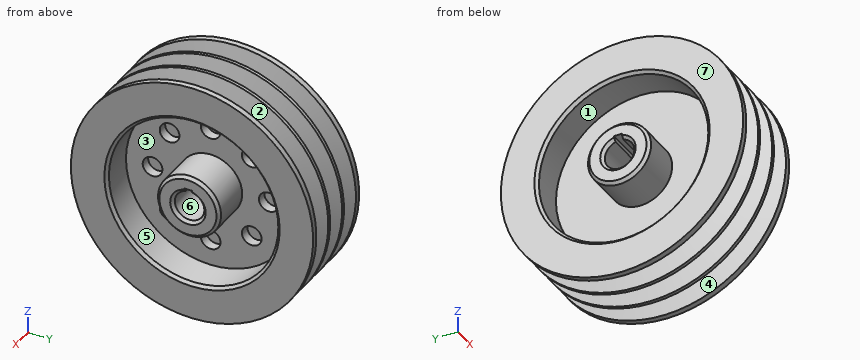
```python
from build123d import *

# Parameters (mm, degrees)
OTHER_START              = -2
OTHER_1_OUTLINE_R        = 10
OTHER_1_DEPTH            = 10
CUT_EXTRUDE_1_DEPTH      = 181.991712517
CUT_EXTRUDE_1_DEPTH_BACK = 181.991712517
SKETCH_4_W               = 24.82633163
SKETCH_4_H               = 8


# Read off the part's stored shape, not the designer's step: 孔1
with BuildPart() as part:
    # 草图1 → 旋转9 (revolve)
    with BuildSketch(Plane.XY, mode=Mode.PRIVATE) as revolve_9_sk:
        Polygon((-47, 15), (47, 15), (50, 18), (50, 29), (47, 32), (8, 32), (8, 86), (39.5, 86), (42.5, 89), (42.5, 123), (36.528653407, 123), (31.178366482, 105.5), (19.821633518, 105.5), (14.471346593, 123), (11.028653407, 123), (5.678366482, 105.5), (-5.678366482, 105.5), (-11.028653407, 123), (-14.471346593, 123), (-19.821633518, 105.5), (-31.178366482, 105.5), (-36.528653407, 123), (-42.5, 123), (-42.5, 89), (-39.5, 86), (-8, 86), (-8, 32), (-47, 32), (-50, 29), (-50, 18), align=None)
    revolve(revolve_9_sk.sketch.rotate(Axis((-111.724769182, 0, 0), (1, 0, 0)), 90), axis=Axis((-111.724769182, 0, 0), (1, 0, 0)))

    # 孔1 outline → 孔1 (cut)
    with BuildSketch(Plane.YZ.offset(OTHER_START)):
        with Locations((0, -59)):
            Circle(OTHER_1_OUTLINE_R)
        with Locations((-41.71930009, -41.71930009)):
            Circle(OTHER_1_OUTLINE_R)
        with Locations((-59, 0)):
            Circle(OTHER_1_OUTLINE_R)
        with Locations((-41.71930009, 41.71930009)):
            Circle(OTHER_1_OUTLINE_R)
        with Locations((0, 59)):
            Circle(OTHER_1_OUTLINE_R)
        with Locations((41.71930009, 41.71930009)):
            Circle(OTHER_1_OUTLINE_R)
        with Locations((59, 0)):
            Circle(OTHER_1_OUTLINE_R)
        with Locations((41.71930009, -41.71930009)):
            Circle(OTHER_1_OUTLINE_R)
    extrude(amount=OTHER_1_DEPTH, mode=Mode.SUBTRACT)

    # 草图4 → 切除-拉伸1 (cut, two sides: drawn at the far end of the back side and taken through both)
    with BuildSketch(Plane(origin=(0, 0, 0), x_dir=(0, 0, -1), z_dir=(1, 0, 0)).offset(-CUT_EXTRUDE_1_DEPTH_BACK)):
        with Locations((-6.586834185, 0)):
            Rectangle(SKETCH_4_W, SKETCH_4_H)
    extrude(amount=CUT_EXTRUDE_1_DEPTH + CUT_EXTRUDE_1_DEPTH_BACK, mode=Mode.SUBTRACT)


solid = part.part
```
Input: part model. Units: mm. Frame: model coordinates. Face numbers are marked on the shaded views. A direction names the side the tool comes from. Coordinates: 2 decimals unless noted, no trailing zeros. Write each loop counter-clockwise with the first axis right and the second up, starting at its lowest first coordinate (ties: lowest second). Pieces come first, ordered by that corner, then holes. Notation, with made-up numbers: M 0,85 L 34,85 A18 ccw 34,108 Z; hole C 61,5.25 d1. An arc over 180 degrees is marked long. Use one line per item in the form item = value.
Q1. Set-up query: the marked faces 1, 2 and 3. Return all of +Z, -Z, +X, -X, +Y, -Y with unobstructed straight access to the full face (end or side cutting, diameter ignored); none if empty.
Answer below:
face_1 = -X
face_2 = none
face_3 = +X
Q2. First-contact query: pin 1 (23 mm diameter, centred on y = 41.72, z = 41.72, fed in from +X); pin 2 (16 mm diameter, centred on y = 0, z = -59, fed in from -X); pin 3 (1.5 mm diameter, centred on x = 3, z = 12.5, fed in from -Y); pin 4 (9 mm diameter, centred on x = -10.5, y = 1, fed in from -Z). Flat tips, straight axial feed; report the tip coordinate or a pass-through.
Answer below:
pin_1 = 8
pin_2 = -8
pin_3 = -104.84
pin_4 = -123
Q3. Section A-A (x = -23). Return loops of the section in (y, z).
Answer below:
outline = C 0,0 d211; C 0,0 d64; hole C 0,0 d172; hole M -4,14.46 A15 ccw long 4,14.46 L 4,19 L -4,19 Z
Q4. Draft query along Y for the marked faces 4, 5, 6 and 7. Return one class per face: released by +Y, released by -Y, zero draft, split by the parting line, or undercut.
Answer below:
face_4 = split by the parting line
face_5 = undercut
face_6 = undercut
face_7 = zero draft
Q5. Material intervals for probe 1 along Z at (x, y) = (-39, 22); probe 2 along X at (y, z) = (-91.5, 78.5); probe 3 along Z at (x, y) = (-4.5, 1.5), sorted ascending. Write a range as from..to.
Answer below:
probe_1 = -121.02..-83.14, -23.24..23.24, 83.14..121.02
probe_2 = -42.5..-35.78, -15.22..-10.28, 10.28..15.22, 35.78..42.5
probe_3 = -105.49..-14.92, 19..105.49
